```python
from build123d import *

# Parameters (mm, degrees)
CROQUIS1_W              = 161
CROQUIS1_H              = 51.5812
SALIENTE_EXTRUIR1_DEPTH = 3
CORTAR_EXTRUIR1_REACH   = 5
CROQUIS2_R              = 1.5
CROQUIS2_R_2            = 4
CORTAR_EXTRUIR2_REACH   = 5
CROQUIS3_R              = 1.5
CORTAR_EXTRUIR3_REACH   = 53.581
CORTAR_EXTRUIR4_DEPTH   = 3
CORTAR_EXTRUIR5_DEPTH   = 10
CORTAR_EXTRUIR6_REACH   = 5
CORTAR_EXTRUIR7_REACH   = 5
CROQUIS11_R             = 1.7
CORTAR_EXTRUIR9_DEPTH   = 10
CORTAR_EXTRUIR10_REACH  = 5


with BuildPart() as part:
    # Croquis1 → Saliente-Extruir1 (new body)
    with BuildSketch(Plane(origin=(0, 0, 0), x_dir=(0, 0, -1), z_dir=(1, 0, 0))):
        Rectangle(CROQUIS1_W, CROQUIS1_H)
    extrude(amount=SALIENTE_EXTRUIR1_DEPTH)

    # Croquis2 → Cortar-Extruir1 (cut, up to next)
    with BuildSketch(Plane(origin=(3, 0, 0), x_dir=(0, 0, -1), z_dir=(1, 0, 0)), mode=Mode.PRIVATE) as cortar_extruir1_sk1:
        with Locations((-75.5, 20.7906)):
            Circle(CROQUIS2_R)
    cortar_extruir1_tool1 = extrude(cortar_extruir1_sk1.sketch, amount=-CORTAR_EXTRUIR1_REACH, mode=Mode.PRIVATE) & part.part
    add(cortar_extruir1_tool1.solids().sort_by_distance((3, 20.7906, 75.5))[0], mode=Mode.SUBTRACT)
    # Croquis2 → Cortar-Extruir1 (cut, up to next)
    with BuildSketch(Plane(origin=(3, 0, 0), x_dir=(0, 0, -1), z_dir=(1, 0, 0)), mode=Mode.PRIVATE) as cortar_extruir1_sk2:
        with Locations((-1.88, 20.7906)):
            Circle(CROQUIS2_R)
    cortar_extruir1_tool2 = extrude(cortar_extruir1_sk2.sketch, amount=-CORTAR_EXTRUIR1_REACH, mode=Mode.PRIVATE) & part.part
    add(cortar_extruir1_tool2.solids().sort_by_distance((3, 20.7906, 1.88))[0], mode=Mode.SUBTRACT)
    # Croquis2 → Cortar-Extruir1 (cut, up to next)
    with BuildSketch(Plane(origin=(3, 0, 0), x_dir=(0, 0, -1), z_dir=(1, 0, 0)), mode=Mode.PRIVATE) as cortar_extruir1_sk3:
        with Locations((-51.5, -3.2094)):
            Circle(CROQUIS2_R_2)
    cortar_extruir1_tool3 = extrude(cortar_extruir1_sk3.sketch, amount=-CORTAR_EXTRUIR1_REACH, mode=Mode.PRIVATE) & part.part
    add(cortar_extruir1_tool3.solids().sort_by_distance((3, -3.2094, 51.5))[0], mode=Mode.SUBTRACT)

    # Croquis3 → Cortar-Extruir2 (cut, up to next)
    with BuildSketch(Plane.ZY, mode=Mode.PRIVATE) as cortar_extruir2_sk1:
        with Locations((-35.801477372, -16.2094)):
            Circle(CROQUIS3_R)
    cortar_extruir2_tool1 = extrude(cortar_extruir2_sk1.sketch, amount=-CORTAR_EXTRUIR2_REACH, mode=Mode.PRIVATE) & part.part
    add(cortar_extruir2_tool1.solids().sort_by_distance((0, -16.2094, -35.801477))[0], mode=Mode.SUBTRACT)

    # Croquis4 → Cortar-Extruir3 (cut, up to next)
    with BuildSketch(Plane(origin=(0, 25.7906, 0), x_dir=(1, 0, 0), z_dir=(0, 1, 0)), mode=Mode.PRIVATE) as cortar_extruir3_sk1:
        Polygon((0, 80.5), (3, 80.5), (3, 58.241825474), (0, 51.808304713), align=None)
    cortar_extruir3_tool1 = extrude(cortar_extruir3_sk1.sketch, amount=-CORTAR_EXTRUIR3_REACH, mode=Mode.PRIVATE) & part.part
    add(cortar_extruir3_tool1.solids().sort_by_distance((1.436864, 25.7906, -67.694835))[0], mode=Mode.SUBTRACT)

    # Croquis5 → Cortar-Extruir4 (cut)
    with BuildSketch(Plane(origin=(3, 0, 0), x_dir=(0, 0, -1), z_dir=(1, 0, 0))):
        Polygon((58.241825474, -25.7906), (58.241825474, -21.2094), (40.910881748, -21.2094), (-11.129087263, -25.7906), align=None)
    extrude(amount=-CORTAR_EXTRUIR4_DEPTH, mode=Mode.SUBTRACT)

    # Croquis6 → Cortar-Extruir5 (cut)
    with BuildSketch(Plane(origin=(3, 0, 0), x_dir=(0, 0, -1), z_dir=(1, 0, 0))):
        Polygon((58.241825474, 25.7906), (38.033287015, 25.7906), (38.033287015, 14.0406), (58.241825474, 2.2906), align=None)
    extrude(amount=-CORTAR_EXTRUIR5_DEPTH, mode=Mode.SUBTRACT)

    # Croquis7 → Cortar-Extruir6 (cut, up to next)
    with BuildSketch(Plane(origin=(3, 0, 0), x_dir=(0, 0, -1), z_dir=(1, 0, 0)), mode=Mode.PRIVATE) as cortar_extruir6_sk1:
        Polygon((38.033287015, 25.7906), (38.033287015, 14.0406), (26.25345467, 25.7906), align=None)
    cortar_extruir6_tool1 = extrude(cortar_extruir6_sk1.sketch, amount=-CORTAR_EXTRUIR6_REACH, mode=Mode.PRIVATE) & part.part
    add(cortar_extruir6_tool1.solids().sort_by_distance((3, 21.873933, -34.106676))[0], mode=Mode.SUBTRACT)

    # Croquis8 → Cortar-Extruir7 (cut, up to next)
    with BuildSketch(Plane(origin=(3, 0, 0), x_dir=(0, 0, -1), z_dir=(1, 0, 0)), mode=Mode.PRIVATE) as cortar_extruir7_sk1:
        Polygon((-38.933678241, -0.034975248), (-35.497792077, -5.986104652), (-28.626019751, -5.986104652), (-25.190133587, -0.034975248), (-28.626019751, 5.916154156), (-35.497792077, 5.916154156), align=None)
    cortar_extruir7_tool1 = extrude(cortar_extruir7_sk1.sketch, amount=-CORTAR_EXTRUIR7_REACH, mode=Mode.PRIVATE) & part.part
    add(cortar_extruir7_tool1.solids().sort_by_distance((3, -0.034975, 32.061906))[0], mode=Mode.SUBTRACT)
    # Croquis8 → Cortar-Extruir7 (cut, up to next)
    with BuildSketch(Plane(origin=(3, 0, 0), x_dir=(0, 0, -1), z_dir=(1, 0, 0)), mode=Mode.PRIVATE) as cortar_extruir7_sk2:
        Polygon((12.785187373, -0.034975248), (8.455060354, 7.465024752), (-0.205193684, 7.465024752), (-4.535320703, -0.034975248), (-0.205193684, -7.534975248), (8.455060354, -7.534975248), align=None)
    cortar_extruir7_tool2 = extrude(cortar_extruir7_sk2.sketch, amount=-CORTAR_EXTRUIR7_REACH, mode=Mode.PRIVATE) & part.part
    add(cortar_extruir7_tool2.solids().sort_by_distance((3, -0.034975, -4.124933))[0], mode=Mode.SUBTRACT)
    # Croquis8 → Cortar-Extruir7 (cut, up to next)
    with BuildSketch(Plane(origin=(3, 0, 0), x_dir=(0, 0, -1), z_dir=(1, 0, 0)), mode=Mode.PRIVATE) as cortar_extruir7_sk3:
        Polygon((29.729088218, 9.284175003), (26.224654714, 12.224743864), (21.925830627, 10.660099854), (21.131440044, 6.154886983), (24.635873548, 3.214318123), (28.934697635, 4.778962133), align=None)
    cortar_extruir7_tool3 = extrude(cortar_extruir7_sk3.sketch, amount=-CORTAR_EXTRUIR7_REACH, mode=Mode.PRIVATE) & part.part
    add(cortar_extruir7_tool3.solids().sort_by_distance((3, 7.719531, -25.430264))[0], mode=Mode.SUBTRACT)
    # Croquis8 → Cortar-Extruir7 (cut, up to next)
    with BuildSketch(Plane(origin=(3, 0, 0), x_dir=(0, 0, -1), z_dir=(1, 0, 0)), mode=Mode.PRIVATE) as cortar_extruir7_sk4:
        Polygon((-19.863794393, -12.020805521), (-15.586299257, -14.846787524), (-11.000179483, -12.555359073), (-10.691554846, -7.437948619), (-14.969049982, -4.611966616), (-19.555169756, -6.903395067), align=None)
    cortar_extruir7_tool4 = extrude(cortar_extruir7_sk4.sketch, amount=-CORTAR_EXTRUIR7_REACH, mode=Mode.PRIVATE) & part.part
    add(cortar_extruir7_tool4.solids().sort_by_distance((3, -9.729377, 15.277675))[0], mode=Mode.SUBTRACT)
    # Croquis8 → Cortar-Extruir7 (cut, up to next)
    with BuildSketch(Plane(origin=(3, 0, 0), x_dir=(0, 0, -1), z_dir=(1, 0, 0)), mode=Mode.PRIVATE) as cortar_extruir7_sk5:
        Polygon((-17.998312172, 9.702211727), (-17.519435903, 5.325448954), (-13.48961002, 3.551786582), (-9.938660407, 6.154886983), (-10.417536677, 10.531649757), (-14.447362559, 12.305312128), align=None)
    cortar_extruir7_tool5 = extrude(cortar_extruir7_sk5.sketch, amount=-CORTAR_EXTRUIR7_REACH, mode=Mode.PRIVATE) & part.part
    add(cortar_extruir7_tool5.solids().sort_by_distance((3, 7.928549, 13.968486))[0], mode=Mode.SUBTRACT)
    # Croquis8 → Cortar-Extruir7 (cut, up to next)
    with BuildSketch(Plane(origin=(3, 0, 0), x_dir=(0, 0, -1), z_dir=(1, 0, 0)), mode=Mode.PRIVATE) as cortar_extruir7_sk6:
        Polygon((30.877634676, -9.772162222), (30.023928106, -4.930551671), (25.404117088, -3.249077972), (21.63801264, -6.409214825), (22.491719211, -11.250825377), (27.111530229, -12.932299075), align=None)
    cortar_extruir7_tool6 = extrude(cortar_extruir7_sk6.sketch, amount=-CORTAR_EXTRUIR7_REACH, mode=Mode.PRIVATE) & part.part
    add(cortar_extruir7_tool6.solids().sort_by_distance((3, -8.090689, -26.257824))[0], mode=Mode.SUBTRACT)
    # Croquis8 → Cortar-Extruir7 (cut, up to next)
    with BuildSketch(Plane(origin=(3, 0, 0), x_dir=(0, 0, -1), z_dir=(1, 0, 0)), mode=Mode.PRIVATE) as cortar_extruir7_sk7:
        Polygon((57.427116401, -0.034975248), (52.689414159, 8.170965745), (43.214009677, 8.170965745), (38.476307436, -0.034975248), (43.214009677, -8.240916241), (52.689414159, -8.240916241), align=None)
    cortar_extruir7_tool7 = extrude(cortar_extruir7_sk7.sketch, amount=-CORTAR_EXTRUIR7_REACH, mode=Mode.PRIVATE) & part.part
    add(cortar_extruir7_tool7.solids().sort_by_distance((3, -0.034975, -47.951712))[0], mode=Mode.SUBTRACT)

    # Croquis11 → Cortar-Extruir9 (cut)
    with BuildSketch(Plane.ZY):
        with Locations((-20.801477372, -16.2094)):
            Circle(CROQUIS11_R)
    extrude(amount=-CORTAR_EXTRUIR9_DEPTH, mode=Mode.SUBTRACT)

    # Croquis12 → Cortar-Extruir10 (cut, up to next)
    with BuildSketch(Plane(origin=(3, 0, 0), x_dir=(0, 0, -1), z_dir=(1, 0, 0)), mode=Mode.PRIVATE) as cortar_extruir10_sk1:
        Polygon((58.241825474, -21.2094), (57.627058446, -16.2094), (40.81163491, -16.2094), (40.81163491, -21.218136931), (40.910881748, -21.2094), align=None)
    cortar_extruir10_tool1 = extrude(cortar_extruir10_sk1.sketch, amount=-CORTAR_EXTRUIR10_REACH, mode=Mode.PRIVATE) & part.part
    add(cortar_extruir10_tool1.solids().sort_by_distance((3, -18.724372, -49.373915))[0], mode=Mode.SUBTRACT)


solid = part.part
```
Design review of the part built by this model. Coordinates are the model's own, in mm. A direction names the side the tool comes from. Coordinates: 2 decimals unless noted, no trailing zeros. Write each loop counter-clockwise with the first axis right and the second up, starting at its lowest first coordinate (ties: lowest second). Pieces come first, ordered by that corner, then holes.
1) Mouldability with a two-part tool opening along Z and no side actions: class faces 3 (the flat face through (1, 0, 80.5)), 4 (the flat face through (0, 6.1, 30)), 5 (the flat face through (1.521, -10.032, 10.848)) as +Z half, -Z half, draft (parallel to the pull), parting line (faces both ways), or undercut.
2) Add section C-C (z = 51.5). Write out the cut boundary in (x, y), plus the area to 3 significant figures.
3) Add section D-D (y = 16). Write out the cut boundary in (x, z).
4) To check wall thickness, follow L1, parallel to Z at x = 1.95, y = -16.5; L2, parallel to Z at x = 1.9, y = 22; L3, parallel to Y at x = 2.25, z = 75.5. State the ranges of each line that lie inside material, in increasing order.
5) Insertion check: pin 1 (13 mm diameter, centred on y = -3.21, z = 51.5, fed in from +X); pin 2 (1.5 mm diameter, centred on x = 1, z = -4, fed in from -Y); pin 3 (2.5 mm diameter, centred on y = 20.79, z = 75.5, fed in from +X); pin 4 (1.5 mm diameter, centred on x = 1, z = -48, fed in from -Y). Each pin has a flat end and moves straight along its axis. Give the tip position at first contact, or say it passes through.
6) Machinability: for faces 1 (the flat face through (1.521, 11.147, -43.01)), 2 (the flat face through (1.5, 4, -26.8)), which of the approach directions +Z, -Z, +X, -X, +Y, -Y give a long, thin tool a straight path to every point of the face, cutting with its end or side? Answer none if there is none.
7) Add section A-A (z = 75.5). Write out the cut boundary in (x, y), plus the area to 3 significant figures.
8) Add section B-B (z = 1.88). Write out the cut boundary in (x, y).
Check result:
1. face 3: +Z half
1. face 4: draft
1. face 5: undercut
2. outline: (0, -25.79) - (3, -25.79) - (3, -7.21) - (0, -7.21) - close; (0, 0.79) - (3, 0.79) - (3, 25.79) - (0, 25.79) - close
2. area: 131 mm2
3. outline: (0, -36.07) - (3, -36.07) - (3, 80.5) - (0, 80.5) - close
4. L1: z = -40.81 to -37.27, -34.33 to -22.48, -19.13 to 80.5
4. L2: z = -30.05 to 0.99, 2.77 to 74.61, 76.39 to 80.5
4. L3: y = -25.79 to 19.29, 22.29 to 25.79
5. pin 1: stops at x = 3
5. pin 2: stops at y = -24.52
5. pin 3: passes through
5. pin 4: stops at y = -16.21
6. face 1: -Z, +X, -X, +Y
6. face 2: +X, -X
7. outline: (0, -25.79) - (3, -25.79) - (3, 19.29) - (0, 19.29) - close; (0, 22.29) - (3, 22.29) - (3, 25.79) - (0, 25.79) - close
7. area: 146 mm2
8. outline: (0, -24.98) - (3, -24.98) - (3, -4.63) - (0, -4.63) - close; (0, 4.56) - (3, 4.56) - (3, 19.29) - (0, 19.29) - close; (0, 22.29) - (3, 22.29) - (3, 25.79) - (0, 25.79) - close
